from build123d import *

# Parameters (mm, degrees)
F1_DEPTH = 111.76
F4_DEPTH = 25.4


with BuildPart() as f1:
    # F0 (on Right) → F1 (new body)
    with BuildSketch(Plane.YZ):
        with BuildLine():
            ThreePointArc((59.190566269, -82.55), (33.2201620113, -41.7067588395), (69.85, -10.0699572513))
            Line((69.85, -10.0699572513), (69.85, 25.8675002325))
            ThreePointArc((69.85, 25.8675002325), (45.4456650544, 50.2718351781), (69.85, 74.6761701237))
            Line((69.85, 74.6761701237), (69.85, 82.55))
            Line((69.85, 82.55), (-69.85, 82.55))
            Line((-69.85, 82.55), (-69.85, -82.55))
            Line((-69.85, -82.55), (59.190566269, -82.55))
        make_face()
        with BuildLine():
            ThreePointArc((59.190566269, -82.55), (91.9419900175, -76.8042285794), (106.8738476743, -47.0938049257))
            ThreePointArc((106.8738476743, -47.0938049257), (96.0298137561, -20.9139911695), (69.85, -10.0699572513))
            Line((69.85, -10.0699572513), (69.85, -16.4199572513))
            ThreePointArc((69.85, -16.4199572513), (91.5396856956, -25.4041192301), (100.5238476743, -47.0938049257))
            ThreePointArc((100.5238476743, -47.0938049257), (91.5396856956, -68.7834906213), (69.85, -77.7676526))
            Line((69.85, -77.7676526), (69.85, -82.55))
            Line((69.85, -82.55), (59.190566269, -82.55))
        make_face()
        with BuildLine():
            Line((69.85, 41.1074995935), (69.85, 25.8675002325))
            ThreePointArc((69.85, 25.8675002325), (87.1064707304, 33.0153644477), (94.2543349456, 50.2718351781))
            ThreePointArc((94.2543349456, 50.2718351781), (87.1064707304, 67.5283059085), (69.85, 74.6761701237))
            Line((69.85, 74.6761701237), (69.85, 59.4361707628))
            ThreePointArc((69.85, 59.4361707628), (76.330163837, 56.7519990151), (79.0143355846, 50.2718351781))
            ThreePointArc((79.0143355846, 50.2718351781), (76.330163837, 43.7916713412), (69.85, 41.1074995935))
        make_face()
        with BuildLine():
            Line((69.85, -16.4199572513), (69.85, -10.0699572513))
            ThreePointArc((69.85, -10.0699572513), (33.2201620113, -41.7067588395), (59.190566269, -82.55))
            Line((59.190566269, -82.55), (69.85, -82.55))
            Line((69.85, -82.55), (69.85, -77.7676526))
            ThreePointArc((69.85, -77.7676526), (39.1761523257, -47.0938049257), (69.85, -16.4199572513))
        make_face()
        with BuildLine():
            ThreePointArc((69.85, 74.6761701237), (45.4456650544, 50.2718351781), (69.85, 25.8675002325))
            Line((69.85, 25.8675002325), (69.85, 41.1074995935))
            ThreePointArc((69.85, 41.1074995935), (60.6856644154, 50.2718351781), (69.85, 59.4361707628))
            Line((69.85, 59.4361707628), (69.85, 74.6761701237))
        make_face()
    extrude(amount=F1_DEPTH)

    # F3 (on face) → F4 (join)
    with BuildSketch(Plane(origin=(0, 0, 0), x_dir=(0, -1, 0), z_dir=(-1, 0, 0))):
        with BuildLine():
            ThreePointArc((39.5199386348, -56.4979792395), (21.8193266657, 4.0562435302), (46.667368415, 62.045038832))
            ThreePointArc((46.667368415, 62.045038832), (-12.2964336182, 6.1132183314), (39.5199386348, -56.4979792395))
        make_face()
        with BuildLine():
            ThreePointArc((25.8455574512, -46.1958609521), (-5.9579445218, 5.7310456276), (31.8542383611, 53.4605458379))
            ThreePointArc((31.8542383611, 53.4605458379), (15.4808375694, 4.438416234), (25.8455574512, -46.1958609521))
        make_face(mode=Mode.SUBTRACT)
    extrude(amount=F4_DEPTH)


solid = f1.part
CAD build for the part. Positions are in the model's coordinates, mm. A direction names the side the tool comes from. Give positions to 0.01 mm unless a question says otherwise; leave off trailing zeros. Order: outer loops, then holes, each group sorted by start corner. A loop starts at its lowest first (then second) coordinate and runs counter-clockwise, first axis right, second up. Notation, with made-up numbers: (45, 31) -> (89, 31) arc R22 ccw to (89, 55) -> close; hole circle Ø1 at (69, 68). An arc over 180 degrees is marked (long way). Return JSON: item names as keys, results as strings.
Q1. Saw through at B-B (z = -30). Write the cut outline in (x, y), then the cut area to 3 significant figures.
Working result:
{"outline": "(-25.4, -26.09) -> (0, -26.09) -> (0, -69.85) -> (111.76, -69.85) -> (111.76, 44.38) -> (0, 44.38) -> (0, 2.73) -> (-25.4, 2.73) -> (-25.4, -5.06) -> (0, -5.06) -> (0, -19.44) -> (-25.4, -19.44) -> close; (0, 95.32) -> (111.76, 95.32) -> (111.76, 102.69) -> (0, 102.69) -> close", "area": "14,000 mm²"}
Q2. Drill centre lines: line 1 (Z direction, x = 49, y = 80); line 2 (Z direction, x = 105, y = 80.5); line 3 (Z direction, x = 77, y = -57.5). Where is each one in solid material? Low to high.
Working result:
{"line 1": "-82.7 to -76.04, -18.15 to -11.49, 28.08 to 72.47", "line 2": "-82.55 to -75.86, -18.33 to -11.63, 28.31 to 72.23", "line 3": "-82.55 to 82.55"}
Q3. Saw through at D-D (y = -2). Write the cut outline in (x, z).
Working result:
{"outline": "(-25.4, -36.29) -> (0, -36.29) -> (0, -82.55) -> (111.76, -82.55) -> (111.76, 82.55) -> (0, 82.55) -> (0, 41.35) -> (-25.4, 41.35) -> (-25.4, 30.67) -> (0, 30.67) -> (0, -25.6) -> (-25.4, -25.6) -> close"}
Q4. Saw through at C-C (y = 55.5). Write the cut outline in (x, z).
Working result:
{"outline": "(0, -82.55) -> (111.76, -82.55) -> (111.76, -74.2) -> (0, -74.2) -> close; (0, -19.98) -> (111.76, -19.98) -> (111.76, 82.55) -> (0, 82.55) -> close"}
Q5. Which spindle directions (+Z, -Z, +X, -X, +Y, -Y) get a long thin tool onto all of the face, cutting with end or side? Do faces 5 (the face through (55, 69.85, 79)), 6 (the face through (-12.52, -21.77, 3.16)), 7 (the face through (55, -6, -82.55)). Say none if no direction does.
Working result:
{"face 5": "+Z, +X, -X, +Y", "face 6": "-X, -Y", "face 7": "-Z, +X, -X, -Y"}
Q6. Flat gauge pins, fed straight in: pin 1 (12 mm diameter, centred on x = 5.5, z = -24, fed in from +Y); pin 2 (5 mm diameter, centred on x = 76.5, y = -19.5, fed in from -Z); pin 3 (2.5 mm diameter, centred on x = 83.5, z = 77, fed in from +Y); pin 4 (3 mm diameter, centred on x = -4, y = -50, fed in from +Z). Where does each tip first touch, or does it go through?
Working result:
{"pin 1": "y = 102.69", "pin 2": "z = -82.55", "pin 3": "y = 69.85", "pin 4": "through"}
Q7. Mould opens along Y. For faces 1 (the face through (55, -69.85, 1)), 2 (the face through (-12.522, -15.528, 5.169)), 3 (the face through (-12.522, 6.005, 4.825)), 4 (the face through (-25.4, -17, 7)) say: pulls with the +Y half, pulls with the -Y half, needs draft (parallel to the pull), parting line crosses it, or undercut.
Working result:
{"face 1": "pulls with the -Y half", "face 2": "undercut", "face 3": "undercut", "face 4": "needs draft"}
Q8. Saw through at A-A (x = 53.5). Write the cut outline in (y, z).
Working result:
{"outline": "(-69.85, -82.55) -> (59.19, -82.55) arc R37.02 ccw (long way) to (69.85, -10.07) -> (69.85, 25.87) arc R24.4 ccw to (69.85, 74.68) -> (69.85, 82.55) -> (-69.85, 82.55) -> close; hole circle Ø61.35 at (69.85, -47.09); hole circle Ø18.33 at (69.85, 50.27)"}
